```python
from build123d import *

# Parameters (mm, degrees)
SKETCH2_R          = 11
CUT_EXTRUDE1_DEPTH = 7


with BuildPart() as part:
    # Sketch1 → Revolve1 (revolve)
    with BuildSketch(Plane.XY):
        with BuildLine():
            Line((0, 9.75), (0, 14.75))
            add(Edge.make_bspline(
                [(24.4, 14.75), (24.4, 36), (12.2, 36), (0, 36), (0, 14.75)],
                knots=[1.570796327, 1.570796327, 1.570796327, 3.141592654, 3.141592654, 4.71238898, 4.71238898, 4.71238898], degree=2, weights=[1, 0.707106781, 1, 0.707106781, 1]))
            Line((24.4, 14.75), (24.4, 9.75))
            Line((24.4, 9.75), (0, 9.75))
        make_face()
    revolve(axis=Axis((0, 0, 0), (1, 0, 0)))

    # Sketch2 → Cut-Extrude1 (cut)
    with BuildSketch(Plane.ZY):
        Circle(SKETCH2_R)
    cut_extrude1 = extrude(amount=-CUT_EXTRUDE1_DEPTH, mode=Mode.SUBTRACT)

    # Mirror1: Cut-Extrude1 across plane
    add(cut_extrude1.mirror(Plane.ZY.offset(-12.2)), mode=Mode.SUBTRACT)


solid = part.part
```
Part model, mm, in its own coordinate system. A direction names the side the tool comes from. Give positions to 0.01 mm unless a question says otherwise; leave off trailing zeros. Use a Markdown table: item, result. Add a question column.
(1) Probe line 1 along Z through (x, y) = (12.5, 0); line 2 along Z through (x, y) = (14.25, -2); line 3 along X through (y, z) = (-10.5, -1). List the from-to ranges inside material, lowest first. Write a range as [from, to].
(2) 3-axis set-ups, long thin cutter, end or side, ignore diameter. For faces 4 (the face through (7, -10, -1)), 5 (the face through (24.4, -6, -10)), 6 (the face through (20.95, -10.74, -2.38)): which of +Z, -Z, +X, -X, +Y, -Y reach the whole face in a straight line?
(3) Drop flat-ended pins along their axis: P1, Ø6, axis at x = 10.5, z = -7.5, coming from the -Y side; P2, Ø3, axis at y = -24, z = -10, coming from the -X side; P3, Ø4, axis at y = 0.5, z = -24, coming from the +X side. Give the stop position or say it passes through.
(4) Mould opens along Y. For faces 1 (the face through (3.45, -10.74, -2.38)), 2 (the face through (17.4, -10, -1)), 3 (the face through (0, 6, -10)) say: +Y half, -Y half, draft (parallel to the pull), parting line (faces both ways), or undercut.
Answer key:
| question | item | result |
|---|---|---|
| 1 | line 1 | [-35.99, -9.75], [9.75, 35.99] |
| 1 | line 2 | [-35.64, -9.54], [9.54, 35.64] |
| 1 | line 3 | [7, 17.4] |
| 2 | face 4 | -X |
| 2 | face 5 | +Z, -Z, +X, +Y, -Y |
| 2 | face 6 | +X |
| 3 | P1 | y = -35.67 |
| 3 | P2 | x = 1.36 |
| 3 | P3 | x = 23.67 |
| 4 | face 1 | undercut |
| 4 | face 2 | undercut |
| 4 | face 3 | draft |
